CAD build for the part. Positions are in the model's coordinates, mm. A direction names the side the tool comes from. Round coordinates to 2 decimals unless told otherwise and drop trailing zeros. Loops run counter-clockwise (first coordinate to the right, second up) from the corner with the lowest first, then second, coordinate; pieces in that order, holes last. Notation, with made-up numbers: M 75,-12 L 128,-12 A25 ccw 128,19 Z; hole C 24,53.25 d9. An arc over 180 degrees is marked long. Use a Markdown table: item, result. Add a question column.
(1) Which spindle directions (+Z, -Z, +X, -X, +Y, -Y) get a long thin tool onto all of the face, cutting with end or side? Do faces 1 (the face through (132.19, 109, 0)), 2 (the face through (128, 107.606, -4)), 3 (the face through (124.88, 120.86, -0.02)). Say none if no direction does.
(2) Wall check: L1, parallel to X at y = 109.25, z = -1; L2, parallel to Y at x = 126, z = -7.5; L3, parallel to Y at x = 130.5, z = -3.25. Give the ranges that are in metal, low to high.
(3) Flat gauge pins, fed straight in: P1, Ø3, axis at x = 127.5, y = 119.5, coming from the -Z side; P2, Ø2, axis at x = 132.5, y = 109.5, coming from the +Z side; P3, Ø2, axis at x = 124, z = 2, coming from the +Y side. Where does each tip first touch, or does it go through?
(4) Two-plate mould, pull along Y, no slides. Class faces 4 (the face through (128, 110.606, 4)), 5 (the face through (124, 99.606, 0)), 6 (the face through (133.185, 124.61, -0.03)), 7 (the face through (124, 109, 9)): released by +Y, released by -Y, zero draft, split by the parting line, or undercut.
(5) Band-saw the part on A-A, the plane y = 103. Write the cut outline in (x, z), and give its area (3 significant figures).
from build123d import *

# Parameters (mm, degrees)
SKETCH_5_OUTSIDE_W  = 26.6
SKETCH_5_OUTSIDE_H  = 26.6
CUT_EXTRUDE_1_DEPTH = 134.94571279


with BuildPart() as part:
    # 草图2 → 旋转1 (revolve)
    with BuildSketch(Plane.XY, mode=Mode.PRIVATE) as revolve_1_sk:
        with BuildLine():
            Line((124.996034131, 120.605813119), (124.189541537, 120.605813119))
            Line((124.189541537, 120.605813119), (124.189541537, 99.605813119))
            Line((124.189541537, 99.605813119), (128.408588613, 99.605813119))
            Line((128.408588613, 99.605813119), (129.189541537, 100.63919496))
            Line((129.189541537, 100.63919496), (129.189541537, 107.605813119))
            Line((129.189541537, 107.605813119), (133.189541537, 107.605813119))
            Line((133.189541537, 107.605813119), (133.189541537, 110.605813119))
            Line((133.189541537, 110.605813119), (128.853577909, 110.605813119))
            ThreePointArc((128.853577909, 110.605813119), (128.024232739, 111.188302984), (128.290749921, 112.166094601))
            ThreePointArc((128.290749921, 112.166094601), (129.689863315, 117.57524199), (124.996034131, 120.605813119))
        make_face()
    revolve(revolve_1_sk.sketch.rotate(Axis((124.189541537, 120.605813119, 0), (0, -1, 0)), 90), axis=Axis((124.189541537, 120.605813119, 0), (0, -1, 0)))

    # 草图5 outside → 切除-拉伸1 (cut, through all)
    with BuildSketch(Plane(origin=(0, 110.605813119, 0), x_dir=(1, 0, 0), z_dir=(0, 1, 0))):
        with Locations((124.19, 0)):
            Rectangle(SKETCH_5_OUTSIDE_W, SKETCH_5_OUTSIDE_H)
        Polygon((124.189541537, 9.237604307), (132.189541537, 4.618802154), (132.189541537, -4.618802154), (124.189541537, -9.237604307), (116.189541537, -4.618802154), (116.189541537, 4.618802154), align=None, mode=Mode.SUBTRACT)
    extrude(amount=-CUT_EXTRUDE_1_DEPTH, mode=Mode.SUBTRACT)

    # 草图6 → 旋转2 (revolve)
    with BuildSketch(Plane.XY, mode=Mode.PRIVATE) as revolve_2_sk:
        with BuildLine():
            Line((133.163968864, 124.631412982), (131.656069582, 126.139312264))
            Line((131.656069582, 126.139312264), (127.824956174, 124.376904464))
            Line((127.824956174, 124.376904464), (127.073314038, 121.958157384))
            ThreePointArc((127.073314038, 121.958157384), (126.655554411, 121.564442646), (126.102557912, 121.718485734))
            Line((126.102557912, 121.718485734), (124.8176438, 123.003399846))
            Line((124.8176438, 123.003399846), (123.778101502, 121.963857549))
            Line((123.778101502, 121.963857549), (127.137257467, 118.604701585))
            Line((127.137257467, 118.604701585), (133.163968864, 124.631412982))
        make_face()
    revolve(revolve_2_sk.sketch.rotate(Axis((124.555886728, 116.023330846, 0), (0.7071067811865461, 0.707106781186549, 0)), 180), axis=Axis((124.555886728, 116.023330846, 0), (0.7071067811865461, 0.707106781186549, 0)))


solid = part.part
Return value:
| question | item | result |
|---|---|---|
| 1 | face 1 | +Z, -Z, +X, -Y |
| 1 | face 2 | -Y |
| 1 | face 3 | none |
| 2 | L1 | 116.19 to 132.19 |
| 2 | L2 | 107.61 to 110.61 |
| 2 | L3 | 107.61 to 110.61, 117.07 to 117.32, 120.97 to 122.81 |
| 3 | P1 | z = -4.75 |
| 3 | P2 | z = 5.02 |
| 3 | P3 | y = 122.71 |
| 4 | face 4 | undercut |
| 4 | face 5 | released by -Y |
| 4 | face 6 | released by +Y |
| 4 | face 7 | zero draft |
| 5 | outline | C 124.19,0 d10 |
| 5 | area | 78.5 mm^2 |
